Verification items for this drawing (mm, ordinates from the low corner). Give positions to 0.01 mm unless a question says otherwise; leave off trailing zeros. Loops run counter-clockwise (first coordinate to the right, second up) from the corner with the lowest first, then second, coordinate; pieces in that order, holes last. Notation, with made-up numbers: M 36,62 L 72,62 A35 ccw 72,97 Z; hole C 81,-29 d6. An arc over 180 degrees is marked long. Use a Markdown table: item, result.
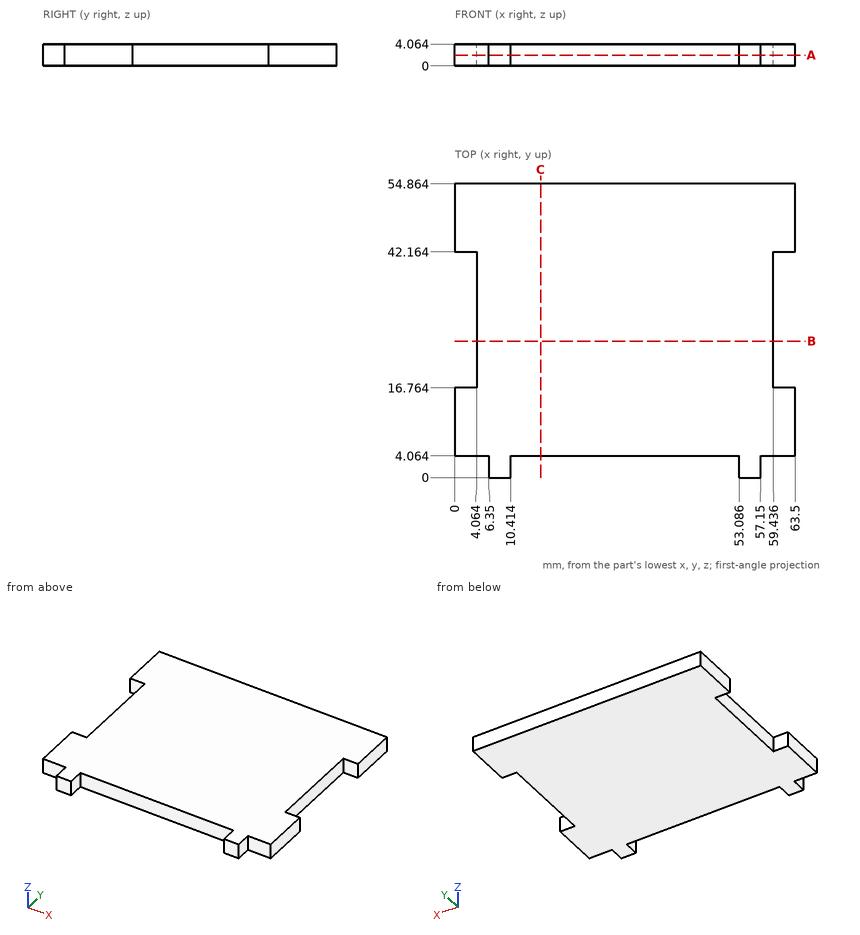
(1) Cross-section at A-A on z = 2. Record the cut outline in (x, y).
Results below:
| item | result |
|---|---|
| outline | M 0,4.06 L 6.35,4.06 L 6.35,0 L 10.41,0 L 10.41,4.06 L 53.09,4.06 L 53.09,0 L 57.15,0 L 57.15,4.06 L 63.5,4.06 L 63.5,16.76 L 59.44,16.76 L 59.44,42.16 L 63.5,42.16 L 63.5,54.86 L 0,54.86 L 0,42.16 L 4.06,42.16 L 4.06,16.76 L 0,16.76 Z |
(2) Cross-section at C-C on x = 16. Record the cut outline in (y, z).
Results below:
| item | result |
|---|---|
| outline | M 4.06,0 L 54.86,0 L 54.86,4.06 L 4.06,4.06 Z |
(3) Gauge pin test, flat ends, axial feed: P1, Ø1, axis at x = 45, z = 2, coming from the -Y side; P2, Ø1.2, axis at y = 2.5, z = 2, coming from the +X side; P3, Ø1.2, axis at y = 24.5, z = 2.5, coming from the -X side. Record the tip position at first contact, or that the pin passes through.
Results below:
| item | result |
|---|---|
| P1 | y = 4.06 |
| P2 | x = 57.15 |
| P3 | x = 4.06 |
(4) Material ranges on line 1 (X direction, y = 2.5, z = 1.35); line 2 (Y direction, x = 60.5, z = 3.05); line 3 (X direction, y = 42, z = 2.55), recorded low to high.
Results below:
| item | result |
|---|---|
| line 1 | 6.35 to 10.41, 53.09 to 57.15 |
| line 2 | 4.06 to 16.76, 42.16 to 54.86 |
| line 3 | 4.06 to 59.44 |
(5) Cross-section at B-B on y = 25.5. Record the cut outline in (x, z), then the cut area to 3 significant figures.
Results below:
| item | result |
|---|---|
| outline | M 4.06,0 L 59.44,0 L 59.44,4.06 L 4.06,4.06 Z |
| area | 225 mm^2 |
